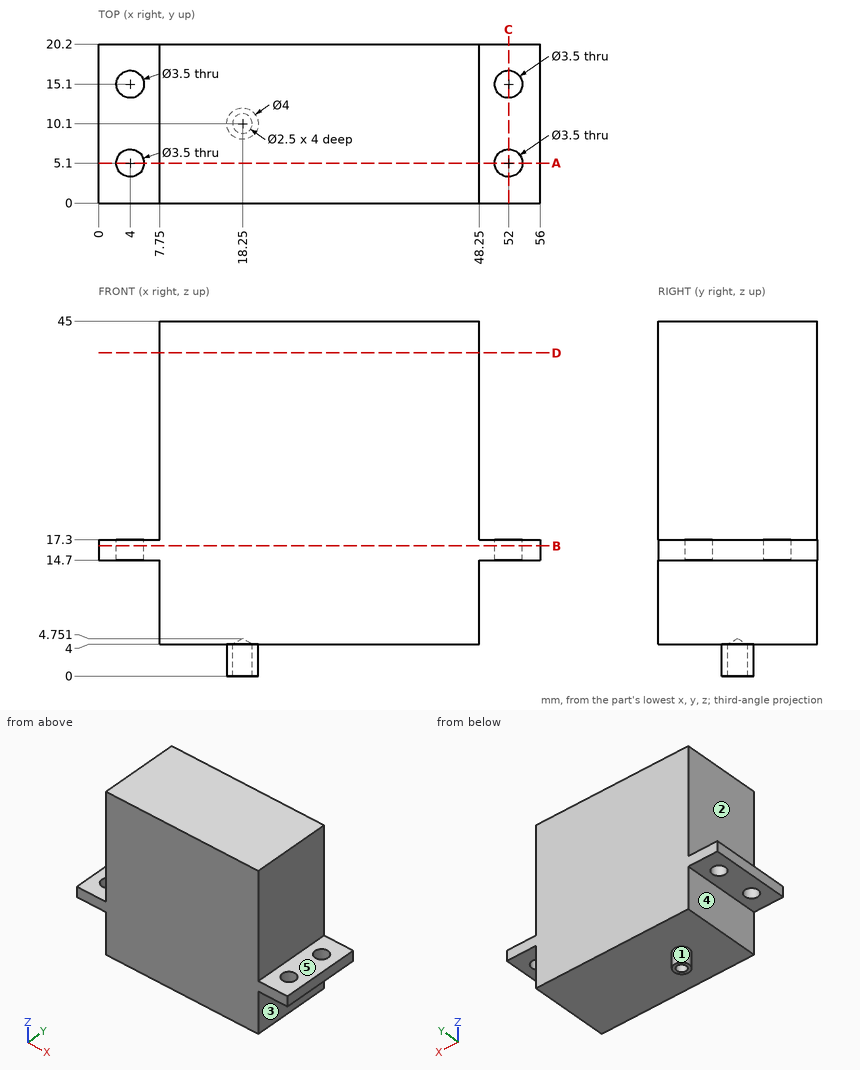
For this review, use the dimensioned drawing (mm, ordinates from the lowest corner) and the shaded views. A direction names the side the tool comes from. Coordinates: 2 decimals unless noted, no trailing zeros. Write each loop counter-clockwise with the first axis right and the second up, starting at its lowest first coordinate (ties: lowest second). Pieces come first, ordered by that corner, then holes. Notation, with made-up numbers: (44, -12.75) -> (49, -12.75) arc R32 cw to (49, 19.25) -> close; hole circle Ø7 at (-6.75, 34.5). An arc over 180 degrees is marked (long way). Write each question's results on one line, items separated by ' | '. Start each with the question number.
(1) Take a section at A-A on y = 5.1. Write out the cut boundary in (x, z), and give its area (3 significant figures).
(2) Clearance check with flat-ended pins moving along their axes: P1, Ø6, axis at y = 15, z = 28, coming from the +X side; P2, Ø3, axis at x = 4, y = 5.1, coming from the +Z side; P3, Ø12, axis at x = 44, y = 4, coming from the -Z side; P4, Ø4, axis at x = 53, y = 8.5, coming from the +Z side. State where each tip first meets the part, or that it passes through.
(3) Take a section at B-B on z = 16.5. Write out the cut boundary in (x, y), and give its area (3 significant figures).
(4) For line 1 along Y through (x, z) = (52, 15); line 2 along Z through (x, y) = (28.5, 7.25); line 3 along X through (y, z) = (8, 10.5), list the stretches that pass through material, from the lowest coordinate up. Write a range as from..to.
(5) Take a section at D-D on z = 41. Write out the cut boundary in (x, y), and give its area (3 significant figures).
(6) Take a section at C-C on x = 52. Write out the cut boundary in (y, z), and give its area (3 significant figures).
(7) Tool access review of the marked faces 1, 2, 3, 4 and 5: name each direction out of +Z, -Z, +X, -X, +Y, -Y from which nothing blocks a thin tool from reaching the whole face with its end or side.
Results found:
1) outline: (0, 14.7) -> (2.25, 14.7) -> (2.25, 17.3) -> (0, 17.3) -> close; (5.75, 14.7) -> (7.75, 14.7) -> (7.75, 4) -> (48.25, 4) -> (48.25, 14.7) -> (50.25, 14.7) -> (50.25, 17.3) -> (48.25, 17.3) -> (48.25, 45) -> (7.75, 45) -> (7.75, 17.3) -> (5.75, 17.3) -> close; (53.75, 14.7) -> (56, 14.7) -> (56, 17.3) -> (53.75, 17.3) -> close | area: 1,680 mm2
2) P1: stops at x = 48.25 | P2: passes through | P3: stops at z = 4 | P4: stops at z = 17.3
3) outline: (0, 0) -> (56, 0) -> (56, 20.2) -> (0, 20.2) -> close; hole circle Ø3.5 at (4, 5.1); hole circle Ø3.5 at (4, 15.1); hole circle Ø3.5 at (52, 5.1); hole circle Ø3.5 at (52, 15.1) | area: 1,090 mm2
4) line 1: y = 0..3.35, 6.85..13.35, 16.85..20.2 | line 2: z = 4..45 | line 3: x = 7.75..48.25
5) outline: (7.75, 0) -> (48.25, 0) -> (48.25, 20.2) -> (7.75, 20.2) -> close | area: 818 mm2
6) outline: (0, 14.7) -> (3.35, 14.7) -> (3.35, 17.3) -> (0, 17.3) -> close; (6.85, 14.7) -> (13.35, 14.7) -> (13.35, 17.3) -> (6.85, 17.3) -> close; (16.85, 14.7) -> (20.2, 14.7) -> (20.2, 17.3) -> (16.85, 17.3) -> close | area: 34.3 mm2
7) face 1: -Z | face 2: +Z, -X, +Y, -Y | face 3: -Z, +X, +Y, -Y | face 4: -Z, -X, +Y, -Y | face 5: +Z, +X, +Y, -Y
